Can you work these out from the model? Positions are in its coordinate system, mm. A direction names the side the tool comes from. Coordinates: 2 decimals unless noted, no trailing zeros. Order: outer loops, then holes, each group sorted by start corner. A loop starts at its lowest first (then second) coordinate and runs counter-clockwise, first axis right, second up. Notation, with made-up numbers: M -23,77 L 19,77 A23 cw 19,105 Z; hole C 38.25,14.5 d9. An arc over 180 degrees is marked long. Answer as a JSON object with one key per item and string values.
from build123d import *

# Parameters (mm, degrees)
FILLET1_R               = 4
CUT_EXTRUDE3_DEPTH      = 106.978541224
CUT_EXTRUDE3_DEPTH_BACK = 106.978541224
SKETCH4_W               = 1.7
SKETCH4_H               = 1.7


with BuildPart() as part:
    # Sketch1 → Revolve1 (revolve)
    with BuildSketch(Plane.XY, mode=Mode.PRIVATE) as revolve1_sk:
        Polygon((0, 0), (10.16, 0), (10.16, 2.5), (3.175, 2.5), (3.175, 105), (0, 105), align=None)
    revolve(revolve1_sk.sketch.rotate(Axis((0, -31.831703756, 0), (0, 1, 0)), 90), axis=Axis((0, -31.831703756, 0), (0, 1, 0)))

    # Fillet1
    fillet1_edges = [part.edges().sort_by_distance(p)[0] for p in [
        (0, 2.5, 3.175),
    ]]
    fillet(fillet1_edges, radius=FILLET1_R)

    # Sketch4 → Cut-Extrude3 (cut, two sides: drawn at the far end of the back side and taken through both)
    with BuildSketch(Plane.XY.offset(-CUT_EXTRUDE3_DEPTH_BACK)):
        with Locations((0, 104.15)):
            Rectangle(SKETCH4_W, SKETCH4_H)
    extrude(amount=CUT_EXTRUDE3_DEPTH + CUT_EXTRUDE3_DEPTH_BACK, mode=Mode.SUBTRACT)


solid = part.part
Item 1: Please list where these lines run through material, in increasing order: line 1 (Z direction, x = 0.25, y = 19.5); line 2 (Y direction, x = -7.5, z = -1.25); line 3 (X direction, y = 6.5, z = 0) (3 decimals).
Answers follow:
{"line 1": "z = -3.17 to 3.17", "line 2": "y = 0 to 2.5", "line 3": "x = -3.175 to 3.175"}
Item 2: Which directions (+Z, -Z, +X, -X, +Y, -Y) give clear straight access to the entire face, cutting with the end or side of a thin tool? Please do faces 1 (the flat face through (0, 103.3, 0)), 2 (the flat face through (-2, 105, 0)), 3 (the flat face through (4, 2.5, -7)).
Answers follow:
{"face 1": "+Z, -Z, +Y", "face 2": "+Z, -Z, +X, -X, +Y", "face 3": "+Y"}
Item 3: I want a section at B-B, the plane y = 86. Write out the boundary of the cut face in (x, z) (3 decimals), plus the area to 3 significant figures.
Answers follow:
{"outline": "C 0,0 d6.35", "area": "31.7 mm^2"}
Item 4: I'm going to push flat-ended pins straight in: pin 1 (6 mm diameter, centred on y = 22.5, z = 3.5, fed in from -X); pin 2 (10 mm diameter, centred on x = 7.5, y = 16.5, fed in from +Z); pin 3 (8 mm diameter, centred on y = 67, z = 3, fed in from -X) (3 decimals). Where does each tip first touch, or does it pass through?
Answers follow:
{"pin 1": "stops at x = -3.14", "pin 2": "stops at z = 1.96", "pin 3": "stops at x = -3.175"}
Item 5: I want a section at A-A, the plane z = 0. Write out the boundary of the cut face in (x, y) (3 decimals).
Answers follow:
{"outline": "M -10.16,0 L 10.16,0 L 10.16,2.5 L 7.175,2.5 A4 cw 3.175,6.5 L 3.175,105 L 0.85,105 L 0.85,103.3 L -0.85,103.3 L -0.85,105 L -3.175,105 L -3.175,6.5 A4 cw -7.175,2.5 L -10.16,2.5 Z"}
Item 6: If we mould it in two halves opening along X, with no side actions, what happens to faces 4 (the flat face through (2, 105, 0)), 5 (the flat face through (0.85, 104, 0)), 6 (the cylindrical face through (1.93, 56.44, 2.52))? For each: pulls with the +X half, pulls with the -X half, needs draft (parallel to the pull), parting line crosses it, or undercut.
Answers follow:
{"face 4": "needs draft", "face 5": "undercut", "face 6": "parting line crosses it"}
